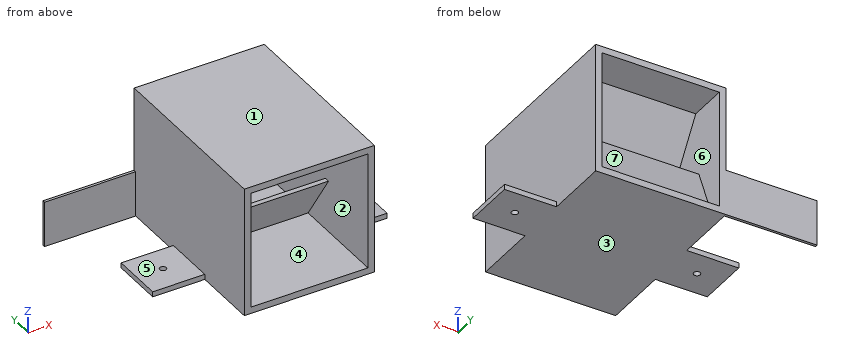
```python
from build123d import *

# Parameters (mm, degrees)
CROQUIS2_W              = 50
CROQUIS2_H              = 50
SALIENTE_EXTRUIR1_DEPTH = 70
CROQUIS3_W              = 45
CROQUIS3_H              = 45
CORTAR_EXTRUIR1_DEPTH   = 130
CROQUIS4_W              = 45
CROQUIS4_H              = 10
SALIENTE_EXTRUIR2_DEPTH = 20
CORTAR_EXTRUIR2_DEPTH   = 45
CROQUIS7_W              = 20
CROQUIS7_H              = 15
SALIENTE_EXTRUIR3_DEPTH = 45
CORTAR_EXTRUIR3_DEPTH   = 45
CROQUIS9_W              = 20
CROQUIS9_H              = 15
SALIENTE_EXTRUIR4_DEPTH = 45
CORTAR_EXTRUIR4_DEPTH   = 45
CROQUIS16_W             = 35
CROQUIS16_H             = 17.5
SALIENTE_EXTRUIR7_DEPTH = 1
CROQUIS17_W             = 20
CROQUIS17_H             = 20
CROQUIS17_R             = 1.25
SALIENTE_EXTRUIR8_DEPTH = 2


with BuildPart() as part:
    # Croquis2 → Saliente-Extruir1 (new body)
    with BuildSketch(Plane(origin=(0, 0, 0), x_dir=(1, 0, 0), z_dir=(0, 1, 0))):
        with Locations((-11.197183099, 3.221830986)):
            Rectangle(CROQUIS2_W, CROQUIS2_H)
    extrude(amount=SALIENTE_EXTRUIR1_DEPTH)

    # Croquis3 → Cortar-Extruir1 (cut)
    with BuildSketch(Plane(origin=(0, 70, 0), x_dir=(1, 0, 0), z_dir=(0, 1, 0))):
        with Locations((-11.197183099, 3.221830986)):
            Rectangle(CROQUIS3_W, CROQUIS3_H)
    extrude(amount=-CORTAR_EXTRUIR1_DEPTH, mode=Mode.SUBTRACT)

    # Croquis4 → Saliente-Extruir2 (add)
    with BuildSketch(Plane.XY.offset(-25.721830986)):
        with Locations((-11.197183099, 60)):
            Rectangle(CROQUIS4_W, CROQUIS4_H)
    extrude(amount=SALIENTE_EXTRUIR2_DEPTH)

    # Croquis5 → Cortar-Extruir2 (cut)
    with BuildSketch(Plane(origin=(-33.697183099, 0, 0), x_dir=(0, 0, -1), z_dir=(1, 0, 0))):
        Polygon((5.721830986, 65), (25.721830986, 65), (5.721830986, 57), align=None)
        Polygon((25.721830986, 55), (25.721830986, 63), (5.721830986, 55), align=None)
    extrude(amount=CORTAR_EXTRUIR2_DEPTH, mode=Mode.SUBTRACT)

    # Croquis7 → Saliente-Extruir3 (add)
    with BuildSketch(Plane(origin=(-33.697183099, 0, 0), x_dir=(0, 0, -1), z_dir=(1, 0, 0))):
        with Locations((-9.278169014, 47.5)):
            Rectangle(CROQUIS7_W, CROQUIS7_H)
    extrude(amount=SALIENTE_EXTRUIR3_DEPTH)

    # Croquis8 → Cortar-Extruir3 (cut)
    with BuildSketch(Plane(origin=(-33.697183099, 0, 0), x_dir=(0, 0, -1), z_dir=(1, 0, 0))):
        Polygon((0.721830986, 55), (0.721830986, 42), (-19.278169014, 55), align=None)
        Polygon((0.721830986, 40), (-19.278169014, 40), (-19.278169014, 53), align=None)
    extrude(amount=CORTAR_EXTRUIR3_DEPTH, mode=Mode.SUBTRACT)

    # Croquis9 → Saliente-Extruir4 (add)
    with BuildSketch(Plane(origin=(-33.697183099, 0, 0), x_dir=(0, 0, -1), z_dir=(1, 0, 0))):
        with Locations((15.721830986, 32.5)):
            Rectangle(CROQUIS9_W, CROQUIS9_H)
    extrude(amount=SALIENTE_EXTRUIR4_DEPTH)

    # Croquis10 → Cortar-Extruir4 (cut)
    with BuildSketch(Plane(origin=(-33.697183099, 0, 0), x_dir=(0, 0, -1), z_dir=(1, 0, 0))):
        Polygon((5.721830986, 40), (5.721830986, 27), (25.721830986, 40), align=None)
        Polygon((5.721830986, 25), (25.721830986, 25), (25.721830986, 38), align=None)
    extrude(amount=CORTAR_EXTRUIR4_DEPTH, mode=Mode.SUBTRACT)

    # Croquis16 → Saliente-Extruir7 (add)
    with BuildSketch(Plane(origin=(0, 70, 0), x_dir=(1, 0, 0), z_dir=(0, 1, 0))):
        with Locations((-53.697183099, 19.471830986)):
            Rectangle(CROQUIS16_W, CROQUIS16_H)
    extrude(amount=-SALIENTE_EXTRUIR7_DEPTH)

    # Croquis17 → Saliente-Extruir8 (add)
    # profile 1 of 2: a face of its own
    with BuildSketch(Plane(origin=(0, 0, -28.221830986), x_dir=(-1, 0, 0), z_dir=(0, 0, -1))):
        with Locations((-23.802816901, 35.103644725)):
            Rectangle(CROQUIS17_W, CROQUIS17_H)
        with Locations((-23.802816901, 35.103644725)):
            Circle(CROQUIS17_R, mode=Mode.SUBTRACT)
    # profile 2 of 2: a face of its own
    with BuildSketch(Plane(origin=(0, 0, -28.221830986), x_dir=(-1, 0, 0), z_dir=(0, 0, -1))):
        with Locations((46.197183099, 35.103644725)):
            Rectangle(CROQUIS17_W, CROQUIS17_H)
        with Locations((46.197183099, 35.103644725)):
            Circle(CROQUIS17_R, mode=Mode.SUBTRACT)
    extrude(amount=-SALIENTE_EXTRUIR8_DEPTH)


solid = part.part
```
Input: part model. Units: mm. Frame: model coordinates. Face numbers are marked on the shaded views. A direction names the side the tool comes from. Give positions to 0.01 mm unless a question says otherwise; leave off trailing zeros. Write each loop counter-clockwise with the first axis right and the second up, starting at its lowest first coordinate (ties: lowest second). Pieces come first, ordered by that corner, then holes. Notation, with made-up numbers: (55.5, 71) - (103.5, 71) arc R13 ccw to (103.5, 83) - close; hole circle Ø7 at (32, -12). An arc over 180 degrees is marked (long way). Write item = value, one per line. Start each with the question number.
1. Section query D-D, the plane z = -17. Output: boundary loops of the cut face in (x, y).
2. Section query A-A, the plane y = 7. Output: boundary loops of the cut face in (x, z).
3. Ray query, L1, parallel to Z at x = 9, y = 26.5; L2, parallel to X at y = 20, z = -6; L3, parallel to Z at x = -26.5, y = 16.5. Return the intervals inside material, ascending.
4. First-contact query: pin 1 Ø10 at (x, y) = (21, 36) entering from +Z; pin 2 Ø8 at (y, z) = (23.5, -7.5) entering from -X; pin 3 Ø8 at (y, z) = (23.5, -14.5) entering from +X. Flat tips, straight axial feed; report the tip coordinate or a pass-through.
5. Section query C-C, the plane z = -2. Output: boundary loops of the cut face in (x, y), then the cut area to 3 significant figures.
6. Access query for the marked faces 3, 4, 5, 6 and 7. Directions: +Z, -Z, +X, -X, +Y, -Y. A direction counts if a zero-diameter tool reaches every point of the face in a straight line with its end or side. Return the directions, or none.
7. Section query B-B, the plane x = -14. Output: boundary loops of the cut face in (y, z).
8. Mould query, pull axis X, two halves, no side actions, for the marked faces 1 and 2. Classes: released by +X, released by -X, zero draft, split by the parting line, or undercut.
Check sheet entries:
q1.outline = (-71.2, 69) - (-36.2, 69) - (-36.2, 0) - (-33.7, 0) - (-33.7, 32.33) - (11.3, 32.33) - (11.3, 0) - (13.8, 0) - (13.8, 70) - (11.3, 70) - (11.3, 61.51) - (-33.7, 61.51) - (-33.7, 70) - (-71.2, 70) - close; hole (-33.7, 34.33) - (11.3, 34.33) - (11.3, 59.51) - (-33.7, 59.51) - close
q2.outline = (-36.2, -28.22) - (13.8, -28.22) - (13.8, 21.78) - (-36.2, 21.78) - close; hole (-33.7, -25.72) - (11.3, -25.72) - (11.3, 19.28) - (-33.7, 19.28) - close
q3.L1 = -28.22 to -25.72, -8.03 to -5.72, 19.28 to 21.78
q3.L2 = -36.2 to -33.7, 11.3 to 13.8
q3.L3 = -28.22 to -25.72, 19.28 to 21.78
q4.pin_1 = -26.22
q4.pin_2 = -36.2
q4.pin_3 = 13.8
q5.outline = (-36.2, 0) - (-33.7, 0) - (-33.7, 70) - (-36.2, 70) - close; (11.3, 0) - (13.8, 0) - (13.8, 70) - (11.3, 70) - close
q5.area = 350 mm2
q6.face_3 = -Z, +X, -X, +Y, -Y
q6.face_4 = -Y
q6.face_5 = +Z, -X, -Y
q6.face_6 = none
q6.face_7 = +Y
q7.outline = (0, -28.22) - (70, -28.22) - (70, -25.72) - (65, -25.72) - (57, -5.72) - (55, -5.72) - (63, -25.72) - (40, -25.72) - (27, -5.72) - (25, -5.72) - (38, -25.72) - (0, -25.72) - close; (0, 19.28) - (53, 19.28) - (40, -0.72) - (42, -0.72) - (55, 19.28) - (70, 19.28) - (70, 21.78) - (0, 21.78) - close
q8.face_1 = zero draft
q8.face_2 = undercut
